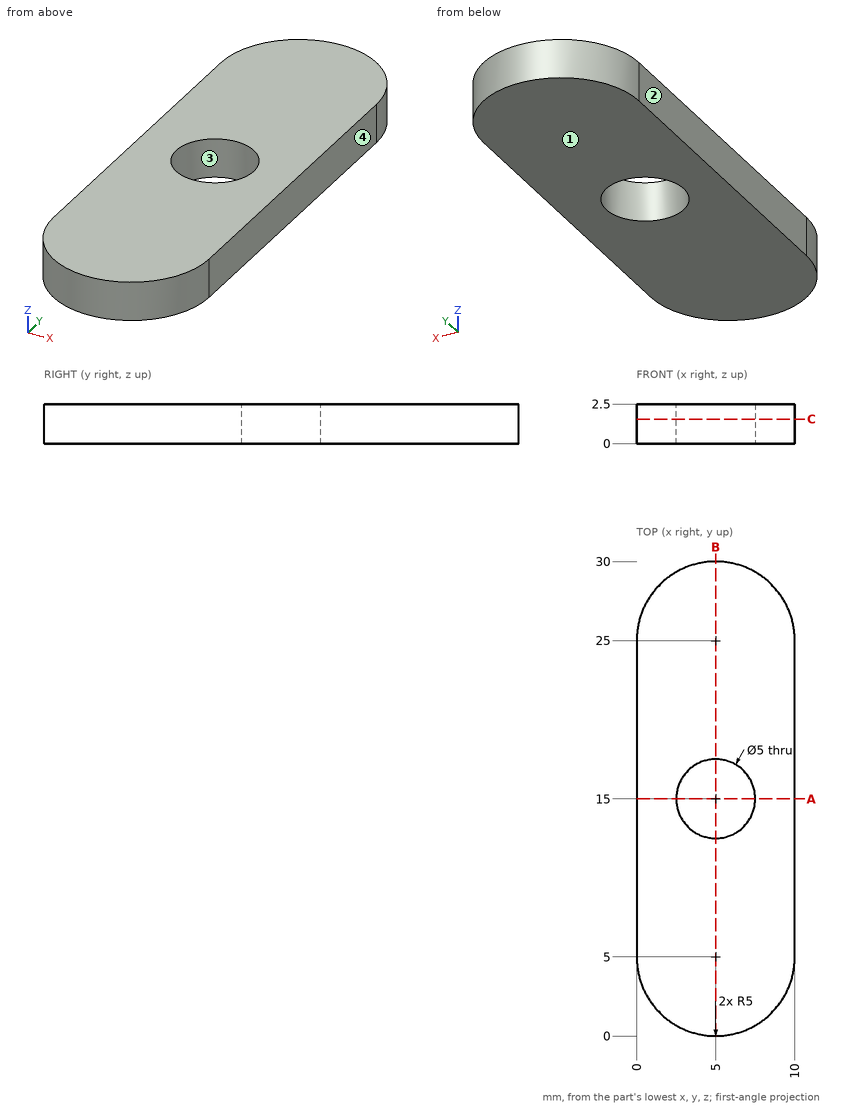
Geometry: see drawing. Coordinates: mm, zero at the bounding-box minimum. Give positions to 0.01 mm unless a question says otherwise; leave off trailing zeros. Loops run counter-clockwise (first coordinate to the right, second up) from the corner with the lowest first, then second, coordinate; pieces in that order, holes last. Notation, with made-up numbers: (-21.5, 48) -> (7.5, 48) arc R25 cw to (7.5, 85) -> close; hole circle Ø3 at (-29.5, 5). An arc over 180 degrees is marked (long way). Use CSV: the item, a comma, the result in double quotes.
(1) Ray query, line 1 along Y through (x, z) = (5, 0.85); line 2 along X through (y, z) = (16, 0.2); line 3 along X through (y, z) = (4, 2.2). Return the intervals inside material, ascending. Write a range as [from, to].
From the geometry:
line 1,"[0, 12.5], [17.5, 30]"
line 2,"[0, 2.71], [7.29, 10]"
line 3,"[0.1, 9.9]"
(2) First-contact query: P1, Ø6, axis at x = 5, y = 15, coming from the +Z side; P2, Ø1.5, axis at x = 3, z = 1.5, coming from the +Y side; P3, Ø1, axis at x = 4, z = 0.5, coming from the -Y side. Flat tips, straight axial feed; report the tip coordinate or a pass-through.
From the geometry:
P1,"z = 2.5"
P2,"y = 29.84"
P3,"y = 0.03"
(3) Cut plane C-C (z = 1.55). Output: boundary loops of the cut face in (x, y), plus the area to 3 significant figures.
From the geometry:
outline,"(0, 5) arc R5 ccw to (10, 5) -> (10, 25) arc R5 ccw to (0, 25) -> close; hole circle Ø5 at (5, 15)"
area,"259 mm^2"
(4) Cut plane B-B (x = 5). Output: boundary loops of the cut face in (y, z).
From the geometry:
outline,"(0, 0) -> (12.5, 0) -> (12.5, 2.5) -> (0, 2.5) -> close; (17.5, 0) -> (30, 0) -> (30, 2.5) -> (17.5, 2.5) -> close"
(5) Pull-direction query (X, two-part tool) for the marked faces 1, 2, 3 and 4; classes: released by +X, released by -X, zero draft, split by the parting line, or undercut.
From the geometry:
face 1,"zero draft"
face 2,"released by -X"
face 3,"undercut"
face 4,"released by +X"
(6) Cut plane A-A (y = 15). Output: boundary loops of the cut face in (x, z).
From the geometry:
outline,"(0, 0) -> (2.5, 0) -> (2.5, 2.5) -> (0, 2.5) -> close; (7.5, 0) -> (10, 0) -> (10, 2.5) -> (7.5, 2.5) -> close"
